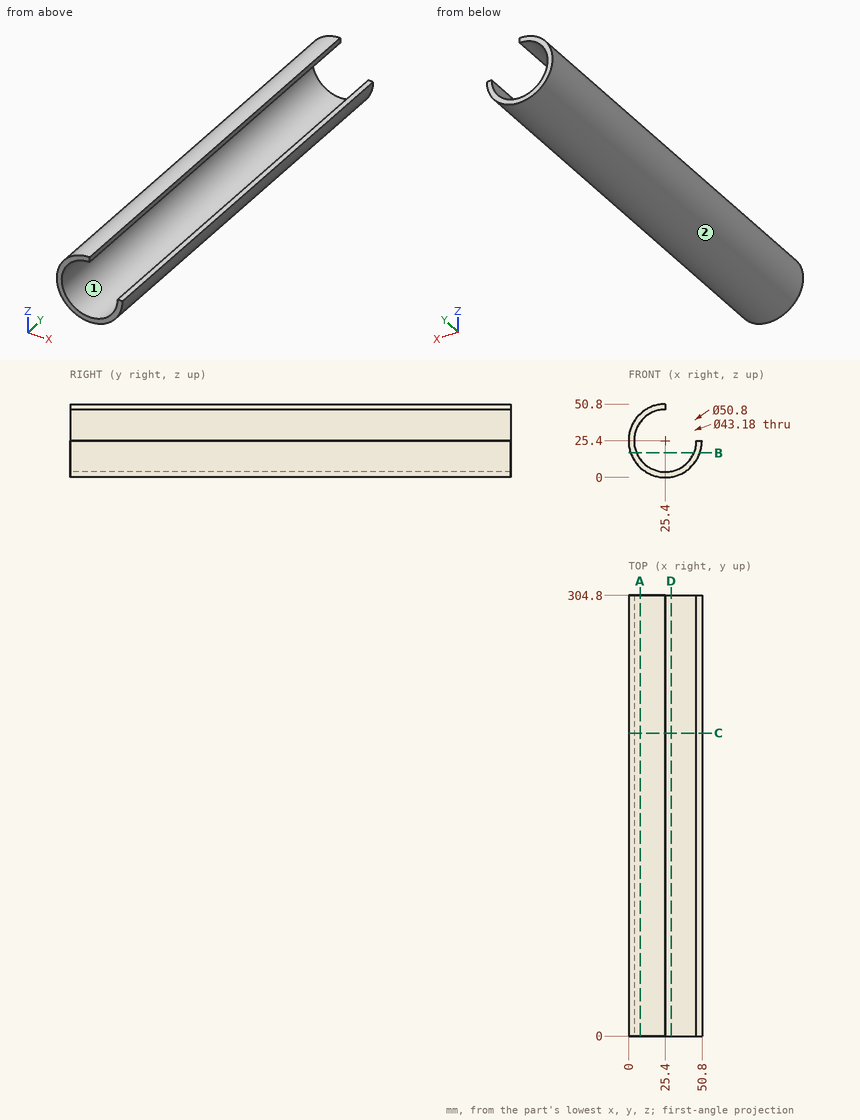
Verification items for this drawing (mm, ordinates from the low corner). Coordinates: 2 decimals unless noted, no trailing zeros. Loops run counter-clockwise (first coordinate to the right, second up) from the corner with the lowest first, then second, coordinate; pieces in that order, holes last. Notation, with made-up numbers: (28.25, 12.5) - (75.25, 12.5) arc R22 cw to (75.25, 41.5) - close; hole circle Ø5 at (53, 74). An arc over 180 degrees is marked (long way). One line per item, written item: value. Start each with the question number.
(1) Cross-section at A-A on x = 8. Enter the section's corners in (y, z).
(2) Mould release check, pull along Z, two halves, no side actions. Record for the marked faces 1 and 2: released by +Z, released by -Z, zero draft, split by the parting line, or undercut.
(3) Cross-section at D-D on x = 29.5. Enter the section's corners in (y, z), plus the area to 3 significant figures.
(4) Depth check by flat-ended pin: P1, Ø4, axis at y = 161.5, z = 49, coming from the +X side; P2, Ø6, axis at x = 31, y = 162.5, coming from the -Z side; P3, Ø1, axis at y = 248, z = 37.5, coming from the +X side; P4, Ø4, axis at x = 24, y = 122, coming from the -Z side. Enter the tip coordinate at first touch or a pass-through.
(5) Cross-section at B-B on z = 17. Enter the section's corners in (x, y).
(6) Cross-section at C-C on y = 209.5. Enter the section's corners in (x, z), plus the area to 3 significant figures.
(7) Material ranges on line 1 (X direction, y = 159, z = 25); line 2 (Z direction, x = 24.5, y = 23.5); line 3 (X direction, y = 151, z = 10), recorded low to high. Write a range as [from, to].
Results below:
1. outline: (0, 6.9) - (304.8, 6.9) - (304.8, 12.62) - (0, 12.62) - close; (0, 38.18) - (304.8, 38.18) - (304.8, 43.9) - (0, 43.9) - close
2. face 1: undercut
2. face 2: split by the parting line
3. outline: (0, 0.33) - (304.8, 0.33) - (304.8, 4.2) - (0, 4.2) - close
3. area: 1,180 mm2
4. P1: stops at x = 25.4
4. P2: stops at z = 0.13
4. P3: stops at x = 7.87
4. P4: stops at z = 0
5. outline: (1.43, 0) - (5.51, 0) - (5.51, 304.8) - (1.43, 304.8) - close; (45.29, 0) - (49.37, 0) - (49.37, 304.8) - (45.29, 304.8) - close
6. outline: (25.4, 46.99) - (25.4, 50.8) arc R25.4 ccw (long way) to (50.8, 25.4) - (46.99, 25.4) arc R21.59 cw (long way) to start
6. area: 422 mm2
7. line 1: x = [0, 3.81], [46.99, 50.8]
7. line 2: z = [0.02, 3.83], [46.97, 50.78]
7. line 3: x = [5.2, 10.27], [40.53, 45.6]
